Here's the drawing with two shaded views (mm, measured from the low corner). I have some questions. A direction names the side the tool comes from. Give positions to 0.01 mm unless a question says otherwise; leave off trailing zeros. Write each loop counter-clockwise with the first axis right and the second up, starting at its lowest first coordinate (ties: lowest second). Pieces come first, ordered by that corner, then holes.
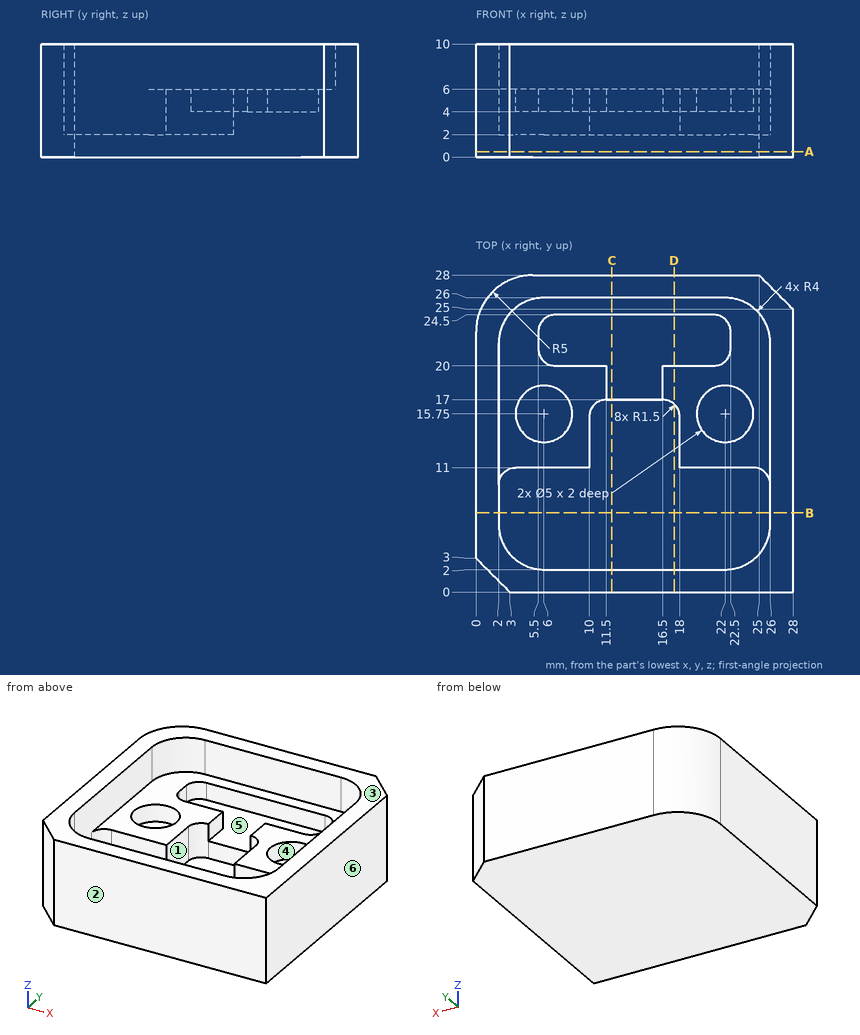
(1) Will these pins go through, and if not, where does the flat tip stop? P1, Ø4.5, axis at x = 6, y = 15.75, coming from the +Z side; P2, Ø1.5, axis at x = 18, y = 11.5, coming from the +Z side.
Returned:
P1: stops at z = 4
P2: stops at z = 6
(2) Imagine slicing it at C-C, the plane x = 12. Write out the boundary of the cut face in (y, z), plus the area to 3 significant figures.
Returned:
outline: (0, 0) - (28, 0) - (28, 10) - (26, 10) - (26, 6) - (24.5, 6) - (24.5, 4) - (17, 4) - (17, 2) - (2, 2) - (2, 10) - (0, 10) - close
area: 109 mm2
(3) If we mould it in two halves opening along X, with no side actions, what happens to the marked faces 3, 4, 5 and 6? For each: +X half, -X half, draft (parallel to the pull), parting line (faces both ways), or undercut.
Returned:
face 3: draft
face 4: undercut
face 5: undercut
face 6: +X half
(4) For the marked faces 1 and 2, which set-ups out of +Z, -Z, +X, -X, +Y, -Y let a thin tool reach every point of the face, with its end or its side?
Returned:
face 1: +Z
face 2: +Z, -Z, +X, -X, -Y
(5) Imagine slicing it at B-B, the plane y = 7. Write out the boundary of the cut face in (x, z), plus the area to 3 significant figures.
Returned:
outline: (0, 0) - (28, 0) - (28, 10) - (26, 10) - (26, 2) - (2, 2) - (2, 10) - (0, 10) - close
area: 88.0 mm2
(6) Imagine slicing it at D-D, the plane x = 17.5. Write out the boundary of the cut face in (y, z).
Returned:
outline: (0, 0) - (28, 0) - (28, 10) - (26, 10) - (26, 6) - (24.5, 6) - (24.5, 4) - (20, 4) - (20, 6) - (16.62, 6) - (16.62, 2) - (2, 2) - (2, 10) - (0, 10) - close
(7) If I drill on L1, parallel to Y at x = 16, z = 2.25; L2, parallel to Y at x = 13, z = 7.5; L3, parallel to Y at x = 22, z = 4.4, over which ranges is the centre line in solid material (lowest first)?
Returned:
L1: y = 0 to 2, 17 to 28
L2: y = 0 to 2, 26 to 28
L3: y = 0 to 2, 11 to 13.25, 18.25 to 20.38, 24.12 to 28
(8) Imagine slicing it at A-A, the plane z = 0.5. Write out the boundary of the cut face in (x, y), plus the area to 3 significant figures.
Returned:
outline: (0, 3) - (3, 0) - (28, 0) - (28, 25) - (25, 28) - (5, 28) arc R5 ccw to (0, 23) - close
area: 770 mm2
